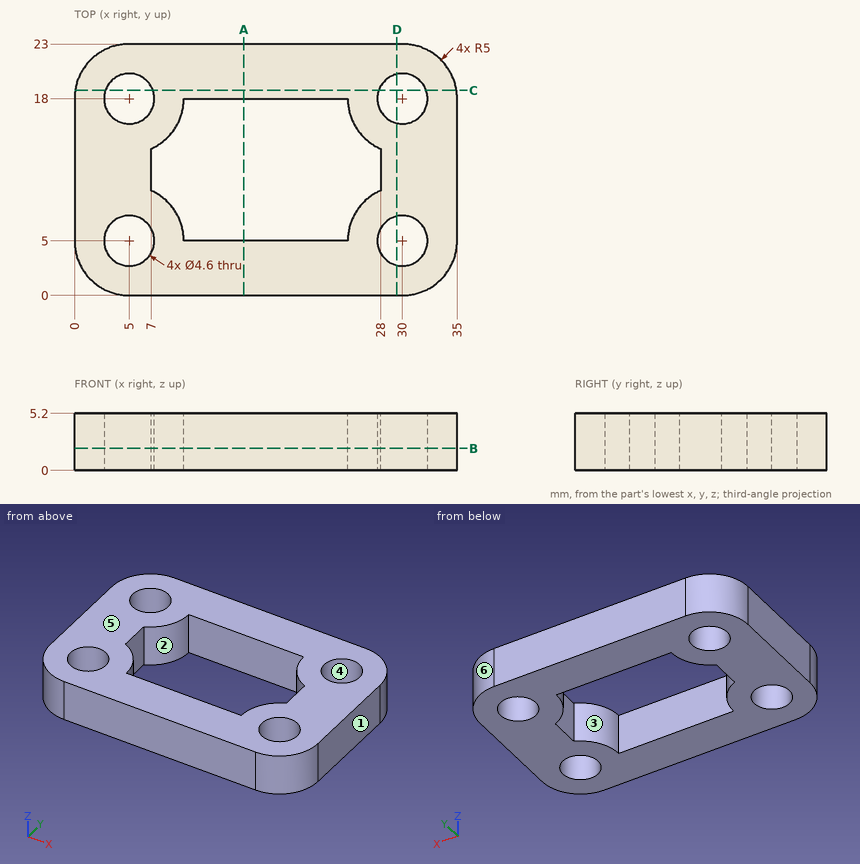
Design review of the part shown in the three views and the two pictorial views. Dimensions are in mm from the part's minimum x, y and z. A direction names the side the tool comes from. Give positions to 0.01 mm unless a question says otherwise; leave off trailing zeros. Loops run counter-clockwise (first coordinate to the right, second up) from the corner with the lowest first, then second, coordinate; pieces in that order, holes last. Notation, with made-up numbers: (58.5, 76.25) -> (110.5, 76.25) arc R24 ccw to (110.5, 105.25) -> close; hole circle Ø6 at (-4.75, 69). An arc over 180 degrees is marked (long way). Write each question's results on one line, items separated by ' | '.
Q1. Wall thickness on L1, parallel to Y at x = 30, z = 2.4; L2, parallel to Y at x = 20, z = 0.6; L3, parallel to X at y = 4.75, z = 2.9: over which ranges is each line inside the solid? List them lowest first.
Reply:
L1: y = 0 to 2.7, 7.3 to 15.7, 20.3 to 23 | L2: y = 0 to 5, 18 to 23 | L3: x = 0.01 to 2.71, 7.29 to 27.71, 32.29 to 34.99
Q2. Take a section at D-D, the plane x = 29.5. Write out the cut boundary in (y, z) (3 decimals).
Reply:
outline: (0, 0) -> (2.755, 0) -> (2.755, 5.2) -> (0, 5.2) -> close; (7.245, 0) -> (15.755, 0) -> (15.755, 5.2) -> (7.245, 5.2) -> close; (20.245, 0) -> (23, 0) -> (23, 5.2) -> (20.245, 5.2) -> close
Q3. Machinability: for the marked faces 1 and 2, which of the approach directions +Z, -Z, +X, -X, +Y, -Y give a long, thin tool a straight path to every point of the face, cutting with its end or side? Answer none if there is none.
Reply:
face 1: +Z, -Z, +X, +Y, -Y | face 2: +Z, -Z
Q4. Take a section at B-B, the plane z = 2. Write out the cut boundary in (x, y).
Reply:
outline: (0, 5) arc R5 ccw to (5, 0) -> (30, 0) arc R5 ccw to (35, 5) -> (35, 18) arc R5 ccw to (30, 23) -> (5, 23) arc R5 ccw to (0, 18) -> close; hole circle Ø4.6 at (5, 5); hole circle Ø4.6 at (5, 18); hole (7, 9.58) arc R5 cw to (10, 5) -> (25, 5) arc R5 cw to (28, 9.58) -> (28, 13.42) arc R5 cw to (25, 18) -> (10, 18) arc R5 cw to (7, 13.42) -> close; hole circle Ø4.6 at (30, 5); hole circle Ø4.6 at (30, 18)
Q5. Take a section at C-C, the plane y = 18.75. Write out the cut boundary in (x, z), plus the area to 3 significant figures.
Reply:
outline: (0.06, 0) -> (2.83, 0) -> (2.83, 5.2) -> (0.06, 5.2) -> close; (7.17, 0) -> (27.83, 0) -> (27.83, 5.2) -> (7.17, 5.2) -> close; (32.17, 0) -> (34.94, 0) -> (34.94, 5.2) -> (32.17, 5.2) -> close | area: 136 mm²
Q6. Take a section at A-A, the plane x = 15.5. Write out the cut boundary in (y, z), plus the area to 3 significant figures.
Reply:
outline: (0, 0) -> (5, 0) -> (5, 5.2) -> (0, 5.2) -> close; (18, 0) -> (23, 0) -> (23, 5.2) -> (18, 5.2) -> close | area: 52.0 mm²
Q7. For pin 1 Ø4 at (x, y) = (30, 5) entering from +Z, flat-tipped, find the tip position at first contact; note if it passes through.
Reply:
pin 1: passes through
Q8. The part is to be moulded in two halves that separate along X. For the marked faces 3, 4, 5 and 6, say which applies: +X half, -X half, draft (parallel to the pull), parting line (faces both ways), or undercut.
Reply:
face 3: undercut | face 4: undercut | face 5: draft | face 6: +X half
